Can you work these out from the model? Positions are in its coordinate system, mm. A direction names the side the tool comes from. Round coordinates to 2 decimals unless told otherwise and drop trailing zeros. Loops run counter-clockwise (first coordinate to the right, second up) from the corner with the lowest first, then second, coordinate; pieces in that order, holes last.
(1) Thinking about a two-plate mould opening in X: for faces 1 (the face through (118, 0, 0)), 2 (the face through (167, -6, 0)), 3 (the face through (78.324, -6.846, -1.52)), which applies, released by +X, released by -X, zero draft, split by the parting line, or undercut?
(2) Which directions (+Z, -Z, +X, -X, +Y, -Y) give clear straight access to the entire face, cutting with the end or side of a thin tool? Please do faces 4 (the face through (0, 0, 0)), 5 (the face through (23, -5, 2)).
(3) I want a section at C-C on x = 159. Write out the boundary of the cut face in (y, z), plus the area to 3 significant figures.
(4) I want a section at A-A on z = 0. Write out the boundary of the cut face in (x, y), plus the area to 3 significant figures.
(5) Will these pins go through, and if not, where does the flat tip stop? pin 1 Ø1 at (y, z) = (0.5, -2.5) entering from +X; pin 2 Ø1 at (x, y) = (116, 5.5) entering from +Z; pin 3 Ø1.5 at (x, z) = (126.5, -3.5) entering from +Y.
(6) If I drill on line 1 along Z through (x, y) = (200, 0.5); line 2 along Y through (x, z) = (145.5, 0); line 3 along Y through (x, z) = (143, 2.25), over which ranges is the centre line in solid material (lowest first)?
from build123d import *

# Parameters (mm, degrees)
F5_START = 118
F4_R     = 6
F5_DEPTH = 102


# Not quite as in the source:
# - a fillet or chamfer that OpenCascade refuses, or shapes differently, is made with other operations: its cross-section is extruded or revolved along the edge and cut away or added


with BuildPart() as f1:
    # F0 (on Front) → F1 (revolve)
    with BuildSketch(Plane.XZ):
        Polygon((0, 5), (0, 0), (218, 0), (218, 9), (130, 9), (26, 5), (26, 7), (23, 7), (23, 5), align=None)
    revolve(axis=Axis((109, 0, 0), (-1, 0, 0)))

    # F2: fillet of radius 2 on 1 edges, made by hand

    # F2_s1 → F2_t2 (revolve)
    with BuildSketch(Plane.XZ):
        with BuildLine():
            ThreePointArc((28.0753312573, 5.079820433), (26.6401911638, 5.6103195704), (26, 7))
            Line((26, 7), (26, 5))
            Line((26, 5), (28.0753312573, 5.079820433))
        make_face()
    revolve(axis=Axis((26, 0, 0), (-1, 0, 0)))

    # F3: chamfer of 0.5 on 3 edges, made by hand

    # F3_s1 → F3_t2 (revolve, cut)
    with BuildSketch(Plane.XZ):
        Polygon((23, 6.5), (23.5, 7), (23, 7), align=None)
    revolve(axis=Axis((23, 0, 0), (-1, 0, 0)), mode=Mode.SUBTRACT)

    # F3_s3 → F3_t4 (revolve, cut)
    with BuildSketch(Plane.XZ):
        Polygon((0, 4.5), (0.5, 5), (0, 5), align=None)
    revolve(axis=Axis((0, 0, 0), (-1, 0, 0)), mode=Mode.SUBTRACT)

    # F3_s5 → F3_t6 (revolve, cut)
    with BuildSketch(Plane.XZ):
        with BuildLine():
            Line((25.5662808863, 7), (26.0527177117, 6.6156685564))
            ThreePointArc((26.0527177117, 6.6156685564), (26.0180191961, 6.799354671), (26, 7))
            Line((26, 7), (25.5662808863, 7))
        make_face()
    revolve(axis=Axis((26, 0, 0), (-1, 0, 0)), mode=Mode.SUBTRACT)

    # F4 (on Right) → F5 (cut)
    with BuildSketch(Plane.YZ.offset(F5_START)):
        Circle(F4_R)
    extrude(amount=F5_DEPTH, mode=Mode.SUBTRACT)


solid = f1.part
Filled sheet:
1. face 1: released by +X
1. face 2: zero draft
1. face 3: undercut
2. face 4: +Z, -Z, -X, +Y, -Y
2. face 5: -X
3. outline: circle Ø18 at (0, 0); hole circle Ø12 at (0, 0)
3. area: 141 mm2
4. outline: (0, -4.5) - (0.5, -5) - (23, -5) - (23, -6.5) - (23.5, -7) - (25.57, -7) - (26.05, -6.62) arc R2 cw to (28.08, -5.08) - (130, -9) - (218, -9) - (218, -6) - (118, -6) - (118, 6) - (218, 6) - (218, 9) - (130, 9) - (28.08, 5.08) arc R2 cw to (26.05, 6.62) - (25.57, 7) - (23.5, 7) - (23, 6.5) - (23, 5) - (0.5, 5) - (0, 4.5) - close
4. area: 2,110 mm2
5. pin 1: stops at x = 118
5. pin 2: stops at z = 6.83
5. pin 3: stops at y = 8.43
6. line 1: z = -8.99 to -5.98, 5.98 to 8.99
6. line 2: y = -9 to -6, 6 to 9
6. line 3: y = -8.71 to -5.56, 5.56 to 8.71
